CAD build for the part. Positions are in the model's coordinates, mm. A direction names the side the tool comes from. Coordinates: 2 decimals unless noted, no trailing zeros. Write each loop counter-clockwise with the first axis right and the second up, starting at its lowest first coordinate (ties: lowest second). Pieces come first, ordered by that corner, then holes. Notation, with made-up numbers: (-14, 42) - (42, 42) arc R31 ccw to (42, 75) - close; hole circle Ø2 at (10, 11). An arc over 180 degrees is marked (long way). One line per question, with ' | ' between items. Start each with the question number.
1. Which spindle directions (+Z, -Z, +X, -X, +Y, -Y) get a long thin tool onto all of the face, cutting with end or side? Do faces 1 (the flat face through (-20, 21, -24)), 2 (the flat face through (26.5, 12, -22)), 3 (the flat face through (40, 8.25, -2)). Say none if no direction does.
2. Probe line 1 (X direction, y = 13.75, z = -9); line 2 (X direction, y = 22.25, z = -38); line 3 (Z direction, x = 1, y = 16.5). List the from-to ranges inside material, lowest first.
3. Two-plate mould, pull along Y, no slides. Class faces 4 (the flat face through (0, 12, -3)), 5 (the cylindrical face through (-52.6, 18.1, -1.5)), 6 (the flat face through (20, 21, -24)): +Y half, -Y half, draft (parallel to the pull), parting line (faces both ways), or undercut.
4. Band-saw the part on D-D, the plane z = -37.5. Write the cut outline in (x, y), then the cut area to 3 significant figures.
5. Flat gauge pins, fed straight in: P1, Ø4, axis at y = 5, z = -24.5, coming from the +X side; P2, Ø0.9, axis at y = 23, z = -19, coming from the -X side; P3, Ø4.5, axis at x = -14, z = -27.5, coming from the -Y side; P4, Ø0.9, axis at x = 36, z = -1.5, coming from the -Y side. Where does each tip first touch, or does it go through?
6. Band-saw the part on A-A, the plane x = -45.5. Write the cut outline in (y, z), then the cut area to 3 significant figures.
7. Band-saw the part on B-B, the plane y = 18. Give the number of separate pieces and of enclosed holes in the cut face, then the cut area to 3 significant figures.
8. Band-saw the part on C-C, the plane x = -8. Write the cut outline in (y, z), then the cut area to 3 significant figures.
from build123d import *

# Parameters (mm, degrees)
BOSS_EXTRUDE5_DEPTH = 24
SKETCH3_W           = 9.5
SKETCH3_H           = 3
BOSS_EXTRUDE7_DEPTH = 42.2
CUT_EXTRUDE3_DEPTH  = 42.2
CUT_EXTRUDE4_DEPTH  = 42.2
FILLET1_R           = 3
FILLET2_R           = 3
FILLET3_R           = 0.5
FILLET4_R           = 0.5
FILLET5_R           = 3
FILLET6_R           = 3
CUT_EXTRUDE5_DEPTH  = 42.2
CUT_EXTRUDE6_DEPTH  = 42.2
CUT_EXTRUDE7_DEPTH  = 42.2
SKETCH8_W           = 47
SKETCH8_H           = 13.670613598
BOSS_EXTRUDE8_DEPTH = 1.5
FILLET7_R           = 10


# Some blends are built 0.0001 mm under size
with BuildPart() as part:
    # Sketch1 → Boss-Extrude5 (new body)
    with BuildSketch(Plane(origin=(0, 0, 0), x_dir=(1, 0, 0), z_dir=(0, 1, 0))):
        Polygon((-55.4, 0), (55.4, 0), (55.4, 3), (26.5, 3), (26.5, 45.2), (21.5, 45.2), (21.5, 3), (-21.5, 3), (-21.5, 45.2), (-26.5, 45.2), (-26.5, 3), (-55.4, 3), align=None)
    extrude(amount=BOSS_EXTRUDE5_DEPTH)

    # Sketch3 → Boss-Extrude7 (add)
    with BuildSketch(Plane(origin=(0, 0, -3), x_dir=(-1, 0, 0), z_dir=(0, 0, -1))):
        with Locations((-16.75, 22.5)):
            Rectangle(SKETCH3_W, SKETCH3_H)
        with Locations((16.75, 22.5)):
            Rectangle(SKETCH3_W, SKETCH3_H)
    extrude(amount=BOSS_EXTRUDE7_DEPTH)

    # Sketch5 → Cut-Extrude3 (cut)
    with BuildSketch(Plane(origin=(0, 21, 0), x_dir=(-1, 0, 0), z_dir=(0, -1, 0))):
        with BuildLine():
            Line((-14.85, 43.490720045), (-14.85, 4.709279955))
            ThreePointArc((-14.85, 4.709279955), (-16.75, 2.809279955), (-18.65, 4.709279955))
            Line((-18.65, 4.709279955), (-18.65, 43.490720045))
            ThreePointArc((-18.65, 43.490720045), (-16.75, 45.390720045), (-14.85, 43.490720045))
        make_face()
    extrude(amount=-CUT_EXTRUDE3_DEPTH, mode=Mode.SUBTRACT)

    # Sketch5<4> → Cut-Extrude4 (cut)
    with BuildSketch(Plane(origin=(0, 21, 0), x_dir=(-1, 0, 0), z_dir=(0, -1, 0))):
        with BuildLine():
            Line((14.85, 4.709279955), (14.85, 43.490720045))
            ThreePointArc((14.85, 43.490720045), (16.75, 45.390720045), (18.65, 43.490720045))
            Line((18.65, 43.490720045), (18.65, 4.709279955))
            ThreePointArc((18.65, 4.709279955), (16.75, 2.809279955), (14.85, 4.709279955))
        make_face()
    extrude(amount=-CUT_EXTRUDE4_DEPTH, mode=Mode.SUBTRACT)

    # Fillet1
    fillet1_edges = [part.edges().sort_by_distance(p)[0] for p in [
        (-26.5, 12, -45.2),
    ]]
    fillet(fillet1_edges, radius=FILLET1_R)

    # Fillet2
    fillet2_edges = [part.edges().sort_by_distance(p)[0] for p in [
        (26.5, 12, -45.2),
    ]]
    fillet(fillet2_edges, radius=FILLET2_R)

    # Fillet3
    fillet3_edges = [part.edges().sort_by_distance(p)[0] for p in [
        (-12, 22.5, -45.2),
    ]]
    fillet(fillet3_edges, radius=FILLET3_R)

    # Fillet4
    fillet4_edges = [part.edges().sort_by_distance(p)[0] for p in [
        (12, 22.5, -45.2),
    ]]
    fillet(fillet4_edges, radius=FILLET4_R)

    # Fillet5
    fillet5_edges = [part.edges().sort_by_distance(p)[0] for p in [
        (55.4, 12, -3),
    ]]
    fillet(fillet5_edges, radius=FILLET5_R - 0.0001)  # a hair under: the kernel refuses the full size

    # Fillet6
    fillet6_edges = [part.edges().sort_by_distance(p)[0] for p in [
        (-55.4, 12, -3),
    ]]
    fillet(fillet6_edges, radius=FILLET6_R - 0.0001)  # a hair under: the kernel refuses the full size

    # Sketch6 → Cut-Extrude5 (cut)
    with BuildSketch(Plane(origin=(0, 0, -3), x_dir=(-1, 0, 0), z_dir=(0, 0, -1))):
        with BuildLine():
            Line((-29.85, 15.25), (-49.05, 15.25))
            ThreePointArc((-49.05, 15.25), (-51.8, 18), (-49.05, 20.75))
            Line((-49.05, 20.75), (-29.85, 20.75))
            ThreePointArc((-29.85, 20.75), (-27.1, 18), (-29.85, 15.25))
        make_face()
        with BuildLine():
            Line((-29.85, 3.75), (-49.05, 3.75))
            ThreePointArc((-49.05, 3.75), (-51.3, 6), (-49.05, 8.25))
            Line((-49.05, 8.25), (-29.85, 8.25))
            ThreePointArc((-29.85, 8.25), (-27.6, 6), (-29.85, 3.75))
        make_face()
    extrude(amount=-CUT_EXTRUDE5_DEPTH, mode=Mode.SUBTRACT)

    # Sketch7 → Cut-Extrude6 (cut)
    with BuildSketch(Plane(origin=(0, 0, -3), x_dir=(-1, 0, 0), z_dir=(0, 0, -1))):
        with BuildLine():
            Line((49.85, 15.25), (29.05, 15.25))
            ThreePointArc((29.05, 15.25), (26.3, 18), (29.05, 20.75))
            Line((29.05, 20.75), (49.85, 20.75))
            ThreePointArc((49.85, 20.75), (52.6, 18), (49.85, 15.25))
        make_face()
    extrude(amount=-CUT_EXTRUDE6_DEPTH, mode=Mode.SUBTRACT)

    # Sketch7<3> → Cut-Extrude7 (cut)
    with BuildSketch(Plane(origin=(0, 0, -3), x_dir=(-1, 0, 0), z_dir=(0, 0, -1))):
        with BuildLine():
            Line((29.05, 7.503040911), (49.85, 7.503040911))
            ThreePointArc((49.85, 7.503040911), (51.85, 5.503040911), (49.85, 3.503040911))
            Line((49.85, 3.503040911), (29.05, 3.503040911))
            ThreePointArc((29.05, 3.503040911), (27.05, 5.503040911), (29.05, 7.503040911))
        make_face()
    extrude(amount=-CUT_EXTRUDE7_DEPTH, mode=Mode.SUBTRACT)

    # Sketch8 → Boss-Extrude8 (add)
    with BuildSketch(Plane(origin=(0, 0, -45.2), x_dir=(-1, 0, 0), z_dir=(0, 0, -1))):
        with Locations((0, 17.164693201)):
            Rectangle(SKETCH8_W, SKETCH8_H)
    extrude(amount=BOSS_EXTRUDE8_DEPTH)

    # Fillet7
    # the kernel refuses this fillet: 10 mm, written as the material it takes off along each edge
    with BuildSketch(Plane(origin=(23.5, 37.169567191, -46.7), x_dir=(0, 0, 1), z_dir=(0, -1, 0)), Plane(origin=(-23.5, -2.840180789, -46.7), x_dir=(0, 0, 1), z_dir=(0, 1, 0))) as fillet7_piece_1:
        with BuildLine():
            CenterArc((10, 5.267826876), FILLET7_R, 180, 31.788330617)
            Line((0, 5.267826876), (-0.2, 5.267826876))
            Line((-0.2, 5.267826876), (-0.2, 0))
            Line((-0.2, 0), (0, -0.2))
            ThreePointArc((0, -0.2), (0.75, -0.2), (1.33, -0.105356538))
            Line((1.33, -0.105356538), (1.5, 0))
        make_face()
    extrude(amount=40.00974798, mode=Mode.SUBTRACT)


solid = part.part
Filled in:
1) face 1: -Y | face 2: -Z, +X, +Y, -Y | face 3: +Z, -Z
2) line 1: x = -26.5 to -21.5, 21.5 to 26.5 | line 2: x = -26.5 to -18.65, -14.85 to -12, 12 to 14.85, 18.65 to 26.5 | line 3: z = -46.7 to -45.2, -3 to 0
3) face 4: draft | face 5: undercut | face 6: -Y half
4) outline: (-26.5, 0) - (-21.5, 0) - (-21.5, 21) - (-18.65, 21) - (-18.65, 24) - (-26.5, 24) - close; (-14.85, 21) - (-12, 21) - (-12, 24) - (-14.85, 24) - close; (12, 21) - (14.85, 21) - (14.85, 24) - (12, 24) - close; (18.65, 21) - (21.5, 21) - (21.5, 0) - (26.5, 0) - (26.5, 24) - (18.65, 24) - close | area: 274 mm²
5) P1: stops at x = 26.5 | P2: stops at x = -26.5 | P3: stops at y = 21 | P4: stops at y = 0
6) outline: (0, -3) - (3.5, -3) - (3.5, 0) - (0, 0) - close; (7.5, -3) - (15.25, -3) - (15.25, 0) - (7.5, 0) - close; (20.75, -3) - (24, -3) - (24, 0) - (20.75, 0) - close | area: 43.5 mm²
7) separate pieces: 3 | enclosed holes: 1 | area: 659 mm²
8) outline: (0, -3) - (24, -3) - (24, 0) - (0, 0) - close; (10.33, -46.7) - (24, -46.7) - (24, -45.2) - (10.33, -45.2) - close | area: 92.5 mm²
